Geometry: final body of the model. Coordinates: model frame, mm. Face numbers are marked on the shaded views. A direction names the side the tool comes from. Give positions to 0.01 mm unless a question says otherwise; leave off trailing zeros. Order: outer loops, then holes, each group sorted by start corner. A loop starts at its lowest first (then second) coordinate and runs counter-clockwise, first axis right, second up. Notation, with made-up numbers: M 31,-36 L 37,-36 A7 ccw 37,-28 Z; hole C 39.5,62 d11. An arc over 180 degrees is marked long. Write item = value, one per line. Start each with the question number.
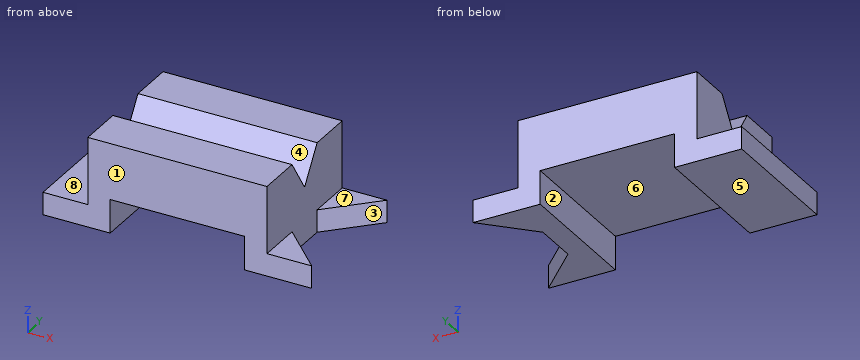
from build123d import *

# Parameters (mm, degrees)
F1_DEPTH = 76.2
F3_DEPTH = 12.7
F5_DEPTH = 152.4


with BuildPart() as f1:
    # F0 (on Front) → F1 (new body)
    with BuildSketch(Plane.XZ):
        Polygon((-38.780687, 0), (-64.180687, 0), (-64.180687, -12.7), (-26.080687, -12.7), (-26.080687, 6.35), (50.119313, 6.35), (50.119313, -12.7), (88.219313, -12.7), (88.219313, 0), (62.819313, 0), (62.819313, 38.1), (50.119313, 38.1), (-38.780687, 38.1), align=None)
    extrude(amount=F1_DEPTH)

    # F2 (on face) → F3 (cut)
    with BuildSketch(Plane.XY):
        Polygon((62.819313, -25.4), (62.819313, -50.8), (88.219313, -76.2), (88.219313, 0), align=None)
    extrude(amount=-F3_DEPTH, mode=Mode.SUBTRACT)

    # F4 (on face) → F5 (cut)
    with BuildSketch(Plane.YZ.offset(62.819313)):
        Polygon((-25.4, 38.1), (-50.8, 38.1), (-38.1, 19.05), align=None)
    extrude(amount=-F5_DEPTH, mode=Mode.SUBTRACT)


solid = f1.part
1) Cut plane C-C (x = -32). Return loops of the section in (y, z).
2) Cut plane A-A (z = 30). Return loops of the section in (x, y).
3) Ray query, L1, parallel to X at y = -39.5, z = 3.5; L2, parallel to X at y = -59, z = 11; L3, parallel to X at y = -25, z = -7.5. Return the intervals inside material, ascending.
4) Draft query along Y for the marked faces 1, 2 and 3. Return one class per face: pulls with the +Y half, pulls with the -Y half, needs draft (parallel to the pull), parting line crosses it, or undercut.
5) Access query for the marked faces 4, 5, 6, 7 and 8. Directions: +Z, -Z, +X, -X, +Y, -Y. A direction counts if a zero-diameter tool reaches every point of the face in a straight line with its end or side. Return the directions, or none.
6) Cut plane B-B (y = -47). Return loops of the section in (x, z), plus the area to 3 significant figures.
7) Cut plane D-D (z = 2). Return loops of the section in (x, y), plus the area to 3 significant figures.
8) Pin query (flat end, axial travel): pin 1 Ø12.5 at (x, y) = (72, -66.5) entering from +Z; pin 2 Ø8 at (y, z) = (-48.5, 16.5) entering from -X; pin 3 Ø21 at (y, z) = (-34.5, -1) entering from +X. Return the tip coordinate at first contact, or that it passes through.
Reply:
q1.outline = M -76.2,-12.7 L 0,-12.7 L 0,38.1 L -25.4,38.1 L -38.1,19.05 L -50.8,38.1 L -76.2,38.1 Z
q2.outline = M -38.78,-76.2 L 62.82,-76.2 L 62.82,-45.4 L -38.78,-45.4 Z; M -38.78,-30.8 L 62.82,-30.8 L 62.82,0 L -38.78,0 Z
q3.L1 = -38.78 to -26.08, 50.12 to 62.82
q3.L2 = -38.78 to 62.82
q3.L3 = -64.18 to -26.08, 50.12 to 63.22
q4.face_1 = pulls with the -Y half
q4.face_2 = needs draft
q4.face_3 = undercut
q5.face_4 = +Z, +X, -X
q5.face_5 = -Z, +X, -X, +Y, -Y
q5.face_6 = -Z, +Y, -Y
q5.face_7 = +Z, +X, +Y, -Y
q5.face_8 = +Z, -X, +Y, -Y
q6.outline = M -64.18,-12.7 L -26.08,-12.7 L -26.08,6.35 L 50.12,6.35 L 50.12,-12.7 L 62.82,-12.7 L 62.82,32.4 L -38.78,32.4 L -38.78,0 L -64.18,0 Z
q6.area = 3,450 mm²
q7.outline = M -38.78,-76.2 L -26.08,-76.2 L -26.08,0 L -38.78,0 Z; M 50.12,-76.2 L 62.82,-76.2 L 62.82,0 L 50.12,0 Z
q7.area = 1,940 mm²
q8.pin_1 = 0
q8.pin_2 = -38.78
q8.pin_3 = 64.22
